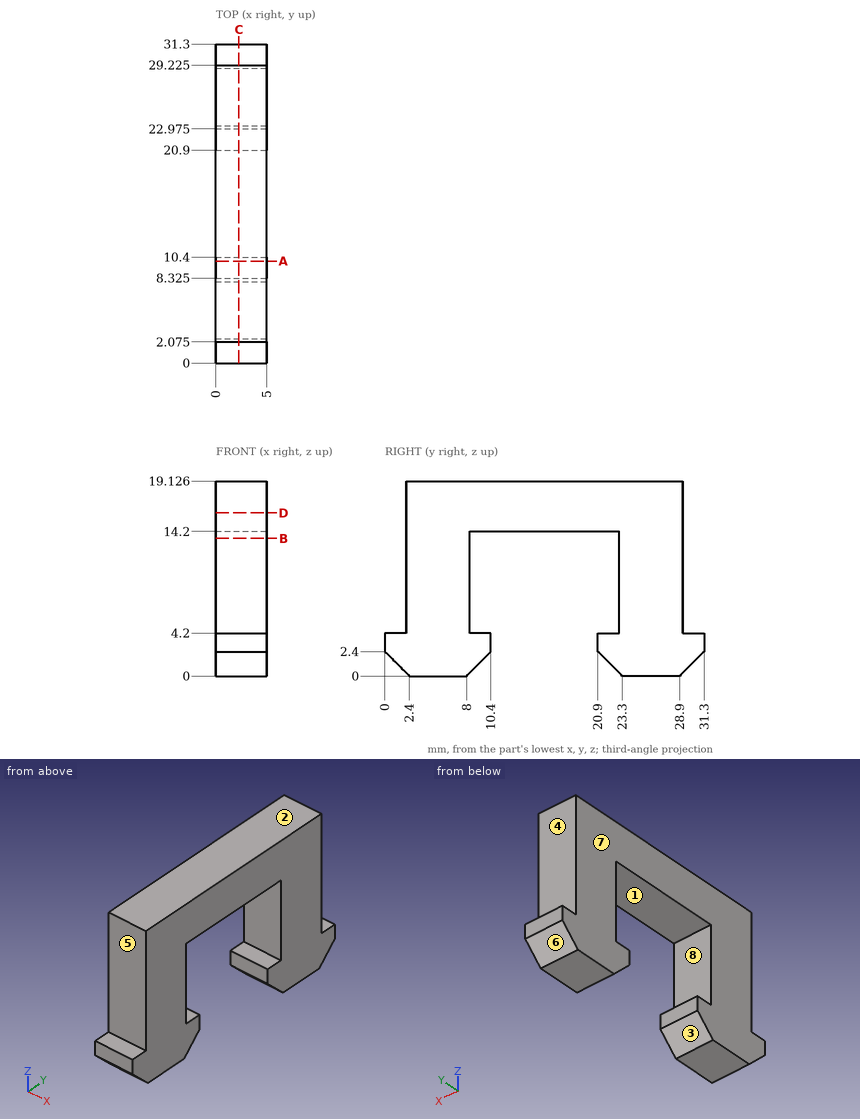
Part print with two shaded views. Sizes in mm from the minimum x, y, z corner. A direction names the side the tool comes from. Coordinates: 2 decimals unless noted, no trailing zeros. Order: outer loops, then holes, each group sorted by start corner. A loop starts at its lowest first (then second) coordinate and runs counter-clockwise, first axis right, second up. Notation, with made-up numbers: (23, -16) - (27, -16) arc R16 ccw to (27, -7) - close; hole circle Ø1 at (-16, -37.5). An arc over 180 degrees is marked (long way). Write item = value, one per line. Start each with the question number.
1) Saw through at B-B on z = 13.5. Write the cut outline in (x, y) (1 decimal).
2) Wall check: line 1 along Y through (x, z) = (1.25, 3.75); line 2 along Y through (x, z) = (1.4, 5.5) (1 decimal); line 3 along Y through (x, z) = (4.5, 16) (1 decimal). Give the ranges that are in metal, low to high. Write a range as from..to.
3) Two-plate mould, pull along Z, no slides. Class the marked faces 6, 7 and 8: pulls with the +Z half, pulls with the -Z half, needs draft (parallel to the pull), parting line crosses it, or undercut.
4) Saw through at C-C on x = 2.25. Write the cut outline in (y, z) (1 decimal).
5) 3-axis set-ups, long thin cutter, end or side, ignore diameter. For the marked faces 1, 2, 3, 4 and 5: which of +Z, -Z, +X, -X, +Y, -Y reach the whole face in a straight line?
6) Saw through at D-D on z = 16. Write the cut outline in (x, y) (1 decimal), then the cut area to 3 significant figures.
7) Saw through at A-A on y = 10. Write the cut outline in (x, z) (1 decimal).
8) Flat gauge pins, fed straight in: pin 1 Ø1 at (x, y) = (1.5, 30.5) entering from +Z; pin 2 Ø1 at (x, z) = (2.5, 16) entering from -Y (3 decimals). Where does each tip first touch, or does it go through?
From the geometry:
q1.outline = (0, 2.1) - (5, 2.1) - (5, 8.3) - (0, 8.3) - close; (0, 23) - (5, 23) - (5, 29.2) - (0, 29.2) - close
q2.line_1 = 0..10.4, 20.9..31.3
q2.line_2 = 2.1..8.3, 23..29.2
q2.line_3 = 2.1..29.2
q3.face_6 = pulls with the -Z half
q3.face_7 = needs draft
q3.face_8 = undercut
q4.outline = (0, 2.4) - (2.4, 0) - (8, 0) - (10.4, 2.4) - (10.4, 4.2) - (8.3, 4.2) - (8.3, 14.2) - (23, 14.2) - (23, 4.2) - (20.9, 4.2) - (20.9, 2.4) - (23.3, 0) - (28.9, 0) - (31.3, 2.4) - (31.3, 4.2) - (29.2, 4.2) - (29.2, 19.1) - (2.1, 19.1) - (2.1, 4.2) - (0, 4.2) - close
q5.face_1 = +X, -X
q5.face_2 = +Z, +X, -X, +Y, -Y
q5.face_3 = -Z, +X, -X
q5.face_4 = +Z, +X, -X, +Y
q5.face_5 = +Z, +X, -X, -Y
q6.outline = (0, 2.1) - (5, 2.1) - (5, 29.2) - (0, 29.2) - close
q6.area = 136 mm^2
q7.outline = (0, 2) - (5, 2) - (5, 4.2) - (0, 4.2) - close; (0, 14.2) - (5, 14.2) - (5, 19.1) - (0, 19.1) - close
q8.pin_1 = 4.2
q8.pin_2 = 2.075
